Design review of the part shown in the three views and the two pictorial views. Dimensions are in mm from the part's minimum x, y and z. A direction names the side the tool comes from. Give positions to 0.01 mm unless a question says otherwise; leave off trailing zeros. Write each loop counter-clockwise with the first axis right and the second up, starting at its lowest first coordinate (ties: lowest second). Pieces come first, ordered by that corner, then holes. Notation, with made-up numbers: (-31, -31) -> (-17, -31) arc R31 ccw to (-17, 0) -> close; hole circle Ø6 at (-40, 24). An arc over 180 degrees is marked (long way). Return JSON: item names as keys, results as strings. Group by question number.
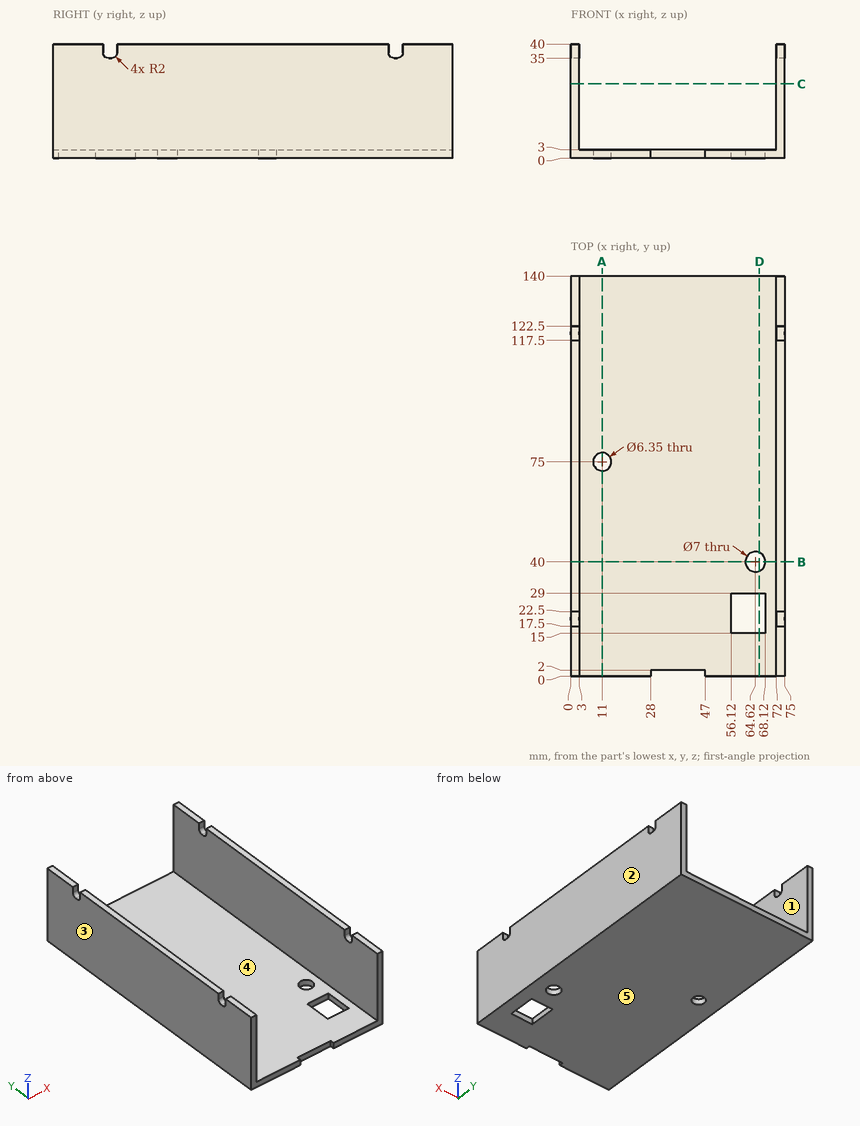
Q1. Mouldability with a two-part tool opening along X and no side actions: class the marked faces 3, 4 and 5 as +X half, -X half, draft (parallel to the pull), parting line (faces both ways), or undercut.
Q2. Take a section at D-D, the plane x = 66. Give the boundary of the cut face in (y, z), plus the area to 3 significant figures.
Q3. Take a section at B-B, the plane y = 40. Give the boundary of the cut face in (x, z).
Q4. Insertion check: pin 1 (5 mm diameter, centred on x = 59.5, y = 84, fed in from +Z); pin 2 (1.1 mm diameter, centred on x = 1, y = 20, fed in from +Z); pin 3 (0.9 mm diameter, centred on x = 37, z = 1, fed in from -Y). Each pin has a flat end and moves straight along its axis. Give the tip position at first contact, or say it passes through.
Q5. For L1, parallel to X at y = 42.5, z = 9.5; L2, parallel to Y at x = 11, z = 1 (3 decimals); L3, parallel to Z at x = 63, y = 123, list the stretches that pass through material, from the lowest coordinate up. Write a range as from..to.
Q6. Tool access review of the marked faces 1 and 2: name each direction out of +Z, -Z, +X, -X, +Y, -Y from which nothing blocks a thin tool from reaching the whole face with its end or side.
Q7. Take a section at A-A, the plane x = 11. Give the boundary of the cut face in (y, z) (3 decimals).
Q8. Take a section at C-C, the plane z = 26. Give the boundary of the cut face in (x, y).
Final values:
{
 "1": {"face 3": "-X half", "face 4": "undercut", "face 5": "draft"},
 "2": {"outline": "(0, 0) -> (15, 0) -> (15, 3) -> (0, 3) -> close; (29, 0) -> (36.78, 0) -> (36.78, 3) -> (29, 3) -> close; (43.22, 0) -> (140, 0) -> (140, 3) -> (43.22, 3) -> close", "area": "359 mm²"},
 "3": {"outline": "(0, 0) -> (61.12, 0) -> (61.12, 3) -> (3, 3) -> (3, 40) -> (0, 40) -> close; (68.12, 0) -> (75, 0) -> (75, 40) -> (72, 40) -> (72, 3) -> (68.12, 3) -> close"},
 "4": {"pin 1": "stops at z = 3", "pin 2": "stops at z = 35", "pin 3": "stops at y = 2"},
 "5": {"L1": "x = 0..3, 72..75", "L2": "y = 0..71.825, 78.175..140", "L3": "z = 0..3"},
 "6": {"face 1": "+Z, +Y, -Y", "face 2": "+Z, -Z, +X, +Y, -Y"},
 "7": {"outline": "(0, 0) -> (71.825, 0) -> (71.825, 3) -> (0, 3) -> close; (78.175, 0) -> (140, 0) -> (140, 3) -> (78.175, 3) -> close"},
 "8": {"outline": "(0, 0) -> (3, 0) -> (3, 140) -> (0, 140) -> close; (72, 0) -> (75, 0) -> (75, 140) -> (72, 140) -> close"}
}
